Autodesk Inventor part; units mm, degrees
ref_plane "Work Plane1" through (63.5, 0, 0) normal (1, 0, 0) x (0, 0, -1)
ref_plane "YZ Plane" through (0, 0, 0) normal (1, 0, 0) x (0, 1, 0)
ref_plane "XZ Plane" through (0, 0, 0) normal (0, 1, 0) x (-1, 0, 0)
sketch "Sketch1" plane through (0, 0, 0) normal (0, 0, 1) x (1, 0, 0)
  line L0 (0, 0) -> (127, 0)
  line L1 (127, 0) -> (127, 25.4)
  line L2 (127, 25.4) -> (0, 25.4)
  line L3 (0, 25.4) -> (0, 0)
  dimension "d0" = 127
  dimension "d1" = 25.4
extrude "Extrusion1" add sketch "Sketch1" along normal blind 6.35
sketch "Sketch2" plane through (0, 0, 6.35) normal (0, 0, 1) x (1, 0, 0)
  line L0 (0, 25.4) -> (0, 0)
  point P0 (12.7, 12.7)
  dimension "d4" = 12.7
hole "Hole1" at (12.7, 12.7, 6.35) direction (0, 0, -1) diameter 6.35 end through all
thread "Thread1"
ref_plane "Work Plane1" through (63.5, 0, 0) normal (1, 0, 0) x (0, 0, -1)
mirror "Mirror1" about plane through (63.5, 0, 0) normal (1, 0, 0) of "Hole1"
thread "Thread2"
sketch "Sketch4" plane through (0, 0, 6.35) normal (0, 0, 1) x (1, 0, 0)
  line L0 (127, 25.4) -> (0, 25.4)
  line L1 (0, 25.4) -> (0, 0)
  line L2 (127, 0) -> (127, 25.4)
  circle A0 centre (50.8, 12.7) radius 1.778
  circle A1 centre (76.2, 12.7) radius 1.778
  dimension "d28" = 12.7
  dimension "d29" = 12.7
  dimension "d30" = 50.8
  dimension "d31" = 50.8
  dimension "d32" = 3.556
extrude "Extrusion3" cut sketch "Sketch4" against normal blind 6.35
properties part number "Plate that doewsn't touch lander"
Check sheet for the modelled part. Datum: model origin and axes. Units: mm. Give positions to 0.01 mm unless a question says otherwise; leave off trailing zeros. Loops run counter-clockwise (first coordinate to the right, second up) from the corner with the lowest first, then second, coordinate; pieces in that order, holes last. Notation, with made-up numbers: (-31, 84.5) - (2, 84.5) arc R14 cw to (2, 106.5) - close; hole circle Ø11 at (47.5, 47.5). An arc over 180 degrees is marked (long way). One line per question, with ' | ' between items. Start each with the question number.
1. Cross-section at C-C, the plane y = 12.7. Enter the section's corners in (x, z) (3 decimals).
2. Cross-section at B-B, the plane z = 1. Enter the section's corners in (x, y) (3 decimals).
3. Cross-section at A-A, the plane x = 114.3. Enter the section's corners in (y, z) (3 decimals).
4. Draft check along Y on faces 1 (the cylindrical face through (49.024, 12.778, 3.219)), 2 (the flat face through (0, 13, 3)), 3 (the flat face through (64, 25.4, 3)), 4 (the cylindrical face through (117.4, 13.39, 3.13)). Enter one of: released by +Y, released by -Y, zero draft, split by the parting line, or undercut.
5. Material ranges on line 1 along Y through (x, z) = (76.2, 2.5); line 2 along Y through (x, z) = (114.3, 1.75) (3 decimals); line 3 along X through (y, z) = (14, 5.75), recorded low to high. Write a range as [from, to].
6. Cross-section at D-D, the plane x = 76.2. Enter the section's corners in (y, z).
Check result:
1) outline: (0, 0) - (9.525, 0) - (9.525, 6.35) - (0, 6.35) - close; (15.875, 0) - (49.022, 0) - (49.022, 6.35) - (15.875, 6.35) - close; (52.578, 0) - (74.422, 0) - (74.422, 6.35) - (52.578, 6.35) - close; (77.978, 0) - (111.125, 0) - (111.125, 6.35) - (77.978, 6.35) - close; (117.475, 0) - (127, 0) - (127, 6.35) - (117.475, 6.35) - close
2) outline: (0, 0) - (127, 0) - (127, 25.4) - (0, 25.4) - close; hole circle Ø6.35 at (12.7, 12.7); hole circle Ø3.556 at (50.8, 12.7); hole circle Ø3.556 at (76.2, 12.7); hole circle Ø6.35 at (114.3, 12.7)
3) outline: (0, 0) - (9.525, 0) - (9.525, 6.35) - (0, 6.35) - close; (15.875, 0) - (25.4, 0) - (25.4, 6.35) - (15.875, 6.35) - close
4) face 1: undercut | face 2: zero draft | face 3: released by +Y | face 4: undercut
5) line 1: y = [0, 10.92], [14.48, 25.4] | line 2: y = [0, 9.525], [15.875, 25.4] | line 3: x = [0, 9.8], [15.6, 49.59], [52.01, 74.99], [77.41, 111.4], [117.2, 127]
6) outline: (0, 0) - (10.92, 0) - (10.92, 6.35) - (0, 6.35) - close; (14.48, 0) - (25.4, 0) - (25.4, 6.35) - (14.48, 6.35) - close
